Part model, mm, in its own coordinate system. A direction names the side the tool comes from. Coordinates: 2 decimals unless noted, no trailing zeros. Loops run counter-clockwise (first coordinate to the right, second up) from the corner with the lowest first, then second, coordinate; pieces in that order, holes last.
```python
from build123d import *

# Parameters (mm, degrees)
BOSS_EXTRUDE1_DEPTH              = 3.175
F_10_0_1935_DIAMETER_HOLE1_D     = 4.9149
F_10_0_1935_DIAMETER_HOLE1_DEPTH = 19.001994
F_10_0_1935_DIAMETER_HOLE1_TIP   = 1.476584928
SKETCH4_R                        = 1.5875
CUT_EXTRUDE1_DEPTH               = 53.937829102
FILLET2_R                        = 35.56
FILLET1_R                        = 6.35


with BuildPart() as part:
    # Sketch1 → Boss-Extrude1 (new body)
    with BuildSketch(Plane(origin=(0, 0, 0), x_dir=(0, 0, -1), z_dir=(1, 0, 0))):
        with BuildLine():
            Line((1.5875, 44.45), (1.5875, 34.925))
            Line((1.5875, 34.925), (-1.5875, 34.925))
            Line((-1.5875, 34.925), (-1.5875, 44.45))
            ThreePointArc((-1.5875, 44.45), (-10.74499019, 41.54249777), (-16.548096362, 33.885007675))
            Line((-16.548096362, 33.885007675), (-28.575, 0))
            Line((-28.575, 0), (-28.575, -12.7))
            Line((-28.575, -12.7), (-14.2875, -12.7))
            Line((-14.2875, -12.7), (-14.2875, 0))
            ThreePointArc((-14.2875, 0), (0, 14.2875), (14.2875, 0))
            Line((14.2875, 0), (14.2875, -12.7))
            Line((14.2875, -12.7), (28.575, -12.7))
            Line((28.575, -12.7), (28.575, 0))
            Line((28.575, 0), (16.548096362, 33.885007675))
            ThreePointArc((16.548096362, 33.885007675), (10.74499019, 41.54249777), (1.5875, 44.45))
        make_face()
    extrude(amount=BOSS_EXTRUDE1_DEPTH)

    # #10 (0.1935) Diameter Hole1
    with Locations(Plane.ZY):
        with Locations((-21.43125, -6.35), (21.43125, -6.35)):
            Hole(F_10_0_1935_DIAMETER_HOLE1_D / 2, depth=F_10_0_1935_DIAMETER_HOLE1_DEPTH)
            with Locations((0, 0, -(F_10_0_1935_DIAMETER_HOLE1_DEPTH + F_10_0_1935_DIAMETER_HOLE1_TIP / 2))):  # 118° drill point
                Cone(0, F_10_0_1935_DIAMETER_HOLE1_D / 2, F_10_0_1935_DIAMETER_HOLE1_TIP, mode=Mode.SUBTRACT)

    # Sketch4 → Cut-Extrude1 (cut, through all)
    with BuildSketch(Plane(origin=(3.175, 0, 0), x_dir=(0, 0, -1), z_dir=(1, 0, 0))):
        with Locations((0, 20.09775)):
            Circle(SKETCH4_R)
        with Locations((-19.048871022, 4.22275)):
            Circle(SKETCH4_R)
        with Locations((19.048871022, 4.22275)):
            Circle(SKETCH4_R)
    extrude(amount=-CUT_EXTRUDE1_DEPTH, mode=Mode.SUBTRACT)

    # Fillet2
    fillet2_edges = [part.edges().sort_by_distance(p)[0] for p in [
        (1.5875, 0, 28.575),
        (1.5875, 0, -28.575),
    ]]
    fillet(fillet2_edges, radius=FILLET2_R)

    # Fillet1
    fillet1_edges = [part.edges().sort_by_distance(p)[0] for p in [
        (1.5875, -12.7, 14.2875),
        (1.5875, -12.7, 28.575),
        (1.5875, -12.7, -28.575),
        (1.5875, -12.7, -14.2875),
    ]]
    fillet(fillet1_edges, radius=FILLET1_R)


solid = part.part
```
Q1. Tool access for faces 4 (the cylindrical face through (1.61, -10.79, 16.1)), 5 (the flat face through (2, 34.925, 0)), 6 (the cylindrical face through (1.565, 41.621, 10.633)): list every direction of +Z, -Z, +X, -X, +Y, -Y with a clear straight run to the whole face (end or side of a thin tool).
Q2. Saw through at A-A (z = 0). List the corners of the cut face in (x, y) (1 decimal).
Q3. Saw through at D-D (z = 7.5). List the corners of the cut face in (x, y) (3 decimals), plus the area to 3 significant figures.
Q4. Mould opens along Y. For faces 1 (the flat face through (1.565, 19.631, -21.607)), 2 (the cylindrical face through (1.565, 14.284, 0.314)), 3 (the cylindrical face through (1.61, 21.44, -0.85)) say: released by +Y, released by -Y, zero draft, split by the parting line, or undercut.
Q5. Drop flat-ended pins along their axis: P1, Ø2.5, axis at y = 4.22, z = 19.05, coming from the -X side; P2, Ø1.5, axis at x = 1.5, z = 10.5, coming from the -Y side; P3, Ø1, axis at x = 2, y = -3.5, coming from the -Z side; P4, Ø1, axis at x = 2.5, y = 19.5, coming from the -Z side. Give the stop position or say it passes through.
Q6. Saw through at B-B (y = 12). List the corners of the cut face in (x, z) (3 decimals), plus the area to 3 significant figures.
Q7. Probe line 1 (Z direction, x = 2.1, y = -5.5); line 2 (Y direction, x = 1.25, z = 0) (1 decimal); line 3 (Z direction, x = 0.9, y = 12). List the from-to ranges inside material, lowest first.
Q8. Saw through at C-C (x = 0.85). Count the separate pieces of the cut face and the enclosed holes in it, plus the area to 3 significant figures.
Checked values:
1. face 4: +X, -X, -Y
1. face 5: +X, -X, +Y
1. face 6: +Z, +X, -X, +Y
2. outline: (0, 14.3) - (3.2, 14.3) - (3.2, 18.5) - (0, 18.5) - close; (0, 21.7) - (3.2, 21.7) - (3.2, 34.9) - (0, 34.9) - close
3. outline: (0, 12.161) - (3.175, 12.161) - (3.175, 43.308) - (0, 43.308) - close
3. area: 98.9 mm2
4. face 1: released by +Y
4. face 2: released by -Y
4. face 3: undercut
5. P1: passes through
5. P2: stops at y = 8.81
5. P3: stops at z = -28.51
5. P4: stops at z = -21.83
6. outline: (0, -24.316) - (3.175, -24.316) - (3.175, -7.755) - (0, -7.755) - close; (0, 7.755) - (3.175, 7.755) - (3.175, 24.316) - (0, 24.316) - close
6. area: 105 mm2
7. line 1: z = -28.57 to -23.74, -19.13 to -14.29, 14.29 to 19.13, 23.74 to 28.57
7. line 2: y = 14.3 to 18.5, 21.7 to 34.9
7. line 3: z = -24.32 to -7.75, 7.75 to 24.32
8. separate pieces: 1
8. enclosed holes: 5
8. area: 1,700 mm2
